Check sheet for the modelled part. Datum: model origin and axes. Units: mm. A direction names the side the tool comes from. Give positions to 0.01 mm unless a question says otherwise; leave off trailing zeros. Write each loop counter-clockwise with the first axis right and the second up, starting at its lowest first coordinate (ties: lowest second). Pieces come first, ordered by that corner, then holes. Notation, with made-up numbers: M 85.5,-20.5 L 108.5,-20.5 A27 ccw 108.5,14.5 Z; hole C -26.75,57 d3. An arc over 180 degrees is marked long. One line per item, written item: value. Start each with the question number.
from build123d import *

# Parameters (mm, degrees)
BOSS_EXTRUDE1_DEPTH = 3
SKETCH2_R           = 4
CUT_EXTRUDE1_DEPTH  = 13
SKETCH3_R           = 1
CUT_EXTRUDE2_DEPTH  = 13
SKETCH4_R           = 1
CUT_EXTRUDE3_DEPTH  = 3
BOSS_EXTRUDE2_DEPTH = 15.5
SKETCH6_R           = 4.6
CUT_EXTRUDE4_DEPTH  = 1.5
SKETCH7_R           = 2
CUT_EXTRUDE5_DEPTH  = 10
SKETCH8_R           = 1
CUT_EXTRUDE6_DEPTH  = 10


with BuildPart() as part:
    # Sketch1 → Boss-Extrude1 (new body)
    with BuildSketch(Plane(origin=(0, 0, 0), x_dir=(1, 0, 0), z_dir=(0, 1, 0))):
        with BuildLine():
            Line((-10, 0), (-14, -25))
            Line((-14, -25), (14, -25))
            Line((14, -25), (10, 0))
            ThreePointArc((10, 0), (0, 10), (-10, 0))
        make_face()
    extrude(amount=BOSS_EXTRUDE1_DEPTH)

    # Sketch2 → Cut-Extrude1 (cut)
    with BuildSketch(Plane(origin=(0, 3, 0), x_dir=(1, 0, 0), z_dir=(0, 1, 0))):
        Circle(SKETCH2_R)
    extrude(amount=-CUT_EXTRUDE1_DEPTH, mode=Mode.SUBTRACT)

    # Sketch3 → Cut-Extrude2 (cut)
    with BuildSketch(Plane(origin=(0, 3, 0), x_dir=(1, 0, 0), z_dir=(0, 1, 0))):
        with Locations((-6.52, -19)):
            Circle(SKETCH3_R)
        with Locations((6.52, -19)):
            Circle(SKETCH3_R)
        with Locations((0, -19)):
            Circle(SKETCH3_R)
    extrude(amount=-CUT_EXTRUDE2_DEPTH, mode=Mode.SUBTRACT)

    # Sketch4 → Cut-Extrude3 (cut)
    with BuildSketch(Plane(origin=(0, 3, 0), x_dir=(1, 0, 0), z_dir=(0, 1, 0))):
        with Locations((0, -7)):
            Circle(SKETCH4_R)
        with Locations((-7, 0)):
            Circle(SKETCH4_R)
        with Locations((0, 7)):
            Circle(SKETCH4_R)
        with Locations((7, 0)):
            Circle(SKETCH4_R)
    extrude(amount=-CUT_EXTRUDE3_DEPTH, mode=Mode.SUBTRACT)

    # Sketch5 → Boss-Extrude2 (add)
    with BuildSketch(Plane(origin=(0, 3, 0), x_dir=(1, 0, 0), z_dir=(0, 1, 0))):
        Polygon((-13.52, -22), (13.52, -22), (14, -25), (-14, -25), align=None)
    extrude(amount=BOSS_EXTRUDE2_DEPTH)

    # Sketch6 → Cut-Extrude4 (cut)
    with BuildSketch(Plane(origin=(0, 3, 0), x_dir=(1, 0, 0), z_dir=(0, 1, 0))):
        Circle(SKETCH6_R)
    extrude(amount=-CUT_EXTRUDE4_DEPTH, mode=Mode.SUBTRACT)

    # Sketch7 → Cut-Extrude5 (cut)
    with BuildSketch(Plane(origin=(0, 3, 0), x_dir=(1, 0, 0), z_dir=(0, 1, 0))):
        with Locations((-7.071067812, 7.071067812)):
            Circle(SKETCH7_R)
        with Locations((7.071067812, 7.071067812)):
            Circle(SKETCH7_R)
    extrude(amount=-CUT_EXTRUDE5_DEPTH, mode=Mode.SUBTRACT)

    # Sketch8 → Cut-Extrude6 (cut)
    with BuildSketch(Plane(origin=(0, 0, 22), x_dir=(-1, 0, 0), z_dir=(0, 0, -1))):
        with Locations((-4.518775135, 7.151837118)):
            Circle(SKETCH8_R)
        with Locations((-4.518775135, 14.651837118)):
            Circle(SKETCH8_R)
        with Locations((9.481224865, 14.651837118)):
            Circle(SKETCH8_R)
        with Locations((9.248832445, 7.151837118)):
            Circle(SKETCH8_R)
    extrude(amount=-CUT_EXTRUDE6_DEPTH, mode=Mode.SUBTRACT)


solid = part.part
1) Gauge pin test, flat ends, axial feed: pin 1 (5 mm diameter, centred on x = 4, z = 8, fed in from +Y); pin 2 (1.6 mm diameter, centred on x = -6.52, z = 19, fed in from -Y); pin 3 (8 mm diameter, centred on x = -8.5, y = 9.5, fed in from -Z). Record the tip position at first contact, or that the pin passes through.
2) Tool access check on faces 1 (the flat face through (-1.7, 1.5, -3.8)), 2 (the cylindrical face through (-6.737, 1.521, 19.976)). Record the directions out of +Z, -Z, +X, -X, +Y, -Y that give a thin tool (end or side, any length) a straight path to the whole face; none if there is none.
3) Cross-section at C-C (z = 3). Record the boundary of the cut face in (x, y).
4) Cross-section at A-A (x = 0). Record the boundary of the cut face in (y, z).
5) Draft check along Y on faces 3 (the cylindrical face through (-9.786, 7.995, 23.479)), 4 (the flat face through (0, 18.5, 23)), 5 (the cylindrical face through (-7.8, 1.5, 0.6)). Enter one of: released by +Y, released by -Y, zero draft, split by the parting line, or undercut.
6) Material ranges on L1, parallel to X at y = 0.75, z = 0; L2, parallel to X at y = 2.6, z = 0; L3, parallel to Z at x = -6.52, y = 0.6, recorded low to high. Write a range as from..to.
7) Cross-section at D-D (x = -6.5). Record the boundary of the cut face in (y, z).
8) Cross-section at B-B (y = 2.25). State how many separate pieces and enclosed holes the cut face has, plus the area to 3 significant figures.
Data:
1. pin 1: stops at y = 3
1. pin 2: passes through
1. pin 3: stops at z = 22
2. face 1: +Y
2. face 2: +Y, -Y
3. outline: M -10.48,0 L -2.65,0 L -2.65,1.5 L -3.49,1.5 L -3.49,3 L -10.48,3 Z; M 2.65,0 L 10.48,0 L 10.48,3 L 3.49,3 L 3.49,1.5 L 2.65,1.5 Z
4. outline: M 0,-10 L 3,-10 L 3,-8 L 0,-8 Z; M 0,-6 L 3,-6 L 3,-4.6 L 1.5,-4.6 L 1.5,-4 L 0,-4 Z; M 0,4 L 1.5,4 L 1.5,4.6 L 3,4.6 L 3,6 L 0,6 Z; M 0,8 L 3,8 L 3,18 L 0,18 Z; M 0,20 L 3,20 L 3,22 L 18.5,22 L 18.5,25 L 0,25 Z
5. face 3: undercut
5. face 4: released by +Y
5. face 5: zero draft
6. L1: x = -10..-8, -6..-4, 4..6, 8..10
6. L2: x = -10..-8, -6..-4.6, 4.6..6, 8..10
6. L3: z = -5.15..-0.88, 0.88..18, 20..25
7. outline: M 0,-5.15 L 3,-5.15 L 3,-0.87 L 0,-0.87 Z; M 0,0.87 L 3,0.87 L 3,18 L 0,18 Z; M 0,20 L 3,20 L 3,22 L 18.5,22 L 18.5,25 L 0,25 Z
8. separate pieces: 1
8. enclosed holes: 8
8. area: 657 mm2
